Work out the finished part from the listing and answer in its coordinate system (mm). Face numbers are marked on the shaded views. Coordinates: 2 decimals unless noted, no trailing zeros. Write each loop counter-clockwise with the first axis right and the second up, starting at its lowest first coordinate (ties: lowest second). Pieces come first, ordered by that corner, then holes. Notation, with made-up numbers: (-13.75, -9.5) - (-0.75, -9.5) arc R10 ccw to (-0.75, -2.5) - close; hole circle Ø6 at (57.25, 21). An arc over 180 degrees is marked (long way). Use one line per item in the form item = value. Start each with the question number.
Item 1: Consider probe 1 along X at (y, z) = (1.1, -38) (3 decimals); probe 2 along Z at (x, y) = (1.5, 2.15); probe 3 along X at (y, z) = (2.2, -36.75). Determine where each line is inside the solid, lowest interval first.
Item 2: Determine the mould class of the marked faces 1, 2 and 3 for opening direction X: released by +X, released by -X, zero draft, split by the parting line, or undercut.
Item 3: A cutting plane is placed at D-D (x = 11). Write down the section's boundary in (y, z), then the cut area to 3 significant figures.
Item 4: A cutting plane is placed at A-A (x = 0). Write down the section's boundary in (y, z) (3 decimals).
Item 5: A cutting plane is placed at C-C (z = -38). Write down the section's boundary in (x, y) (3 decimals), then the cut area to 3 significant figures.
Item 6: A cutting plane is placed at B-B (y = 1.05). Write down the section's boundary in (x, z) (3 decimals).
Item 7: Given pin 1 (1.5 mm diameter, centred on x = 8, y = 2.5, fed in from +Z), flat-ended and moving along its own axis, determine where the tip first touches the part or whether it passes through.
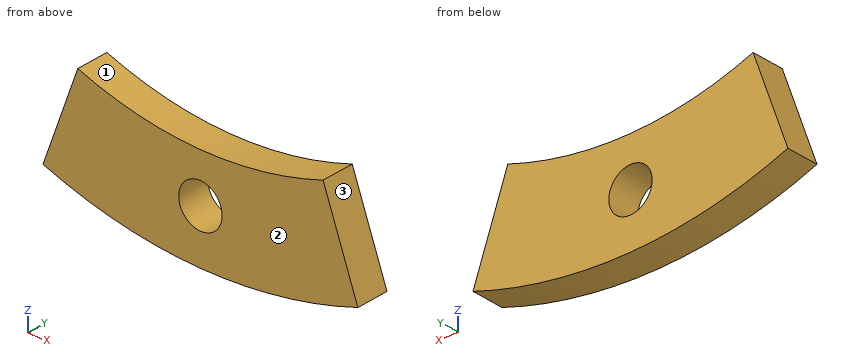
from build123d import *

# Parameters (mm, degrees)
SKETCH1_R               = 43
SKETCH1_R_2             = 33.5
BOSS_EXTRUDE1_DEPTH     = 3
CUT_EXTRUDE1_START      = -4
CUT_EXTRUDE1_DEPTH      = 5
SKETCH3_R               = 2.025
CUT_EXTRUDE2_DEPTH      = 1
CUT_EXTRUDE2_DEPTH_BACK = 4


with BuildPart() as part:
    # Sketch1 → Boss-Extrude1 (new body)
    with BuildSketch(Plane(origin=(0, 0, 0), x_dir=(1, 0, 0), z_dir=(0, 1, 0))):
        Circle(SKETCH1_R)
        Circle(SKETCH1_R_2, mode=Mode.SUBTRACT)
    extrude(amount=BOSS_EXTRUDE1_DEPTH)

    # Sketch2 → Cut-Extrude1 (cut)
    with BuildSketch(Plane(origin=(0, 3, 0), x_dir=(1, 0, 0), z_dir=(0, 1, 0)).offset(CUT_EXTRUDE1_START)):
        with BuildLine():
            Line((0, 0), (0, -52.31984462))
            ThreePointArc((0, -52.31984462), (51.524988618, -9.085245674), (17.894440756, 49.16457191))
            Line((17.894440756, 49.16457191), (0, 0))
        make_face()
    cut_extrude1 = extrude(amount=CUT_EXTRUDE1_DEPTH, mode=Mode.SUBTRACT)

    # Mirror1: Cut-Extrude1 across plane
    add(cut_extrude1.mirror(Plane(origin=(0, 0, 0), x_dir=(0, 0, 1), z_dir=(1, 0, 0))), mode=Mode.SUBTRACT)

    # Sketch3 → Cut-Extrude2 (cut, two sides)
    with BuildSketch(Plane(origin=(0, 3, 0), x_dir=(1, 0, 0), z_dir=(0, 1, 0))) as cut_extrude2_sk:
        with Locations((0, 38)):
            Circle(SKETCH3_R)
    extrude(amount=CUT_EXTRUDE2_DEPTH, mode=Mode.SUBTRACT)
    extrude(cut_extrude2_sk.sketch, amount=-CUT_EXTRUDE2_DEPTH_BACK, mode=Mode.SUBTRACT)


solid = part.part
Answer:
q1.probe_1 = -13.831 to -2.025, 2.025 to 13.831
q1.probe_2 = -42.97 to -39.36, -36.64 to -33.47
q1.probe_3 = -13.38 to -1.59, 1.59 to 13.38
q2.face_1 = undercut
q2.face_2 = zero draft
q2.face_3 = released by +X
q3.outline = (0, -41.57) - (3, -41.57) - (3, -31.64) - (0, -31.64) - close
q3.area = 29.8 mm²
q4.outline = (0, -43) - (3, -43) - (3, -40.025) - (0, -40.025) - close; (0, -35.975) - (3, -35.975) - (3, -33.5) - (0, -33.5) - close
q5.outline = (-13.831, 0) - (-2.025, 0) - (-2.025, 3) - (-13.831, 3) - close; (2.025, 0) - (13.831, 0) - (13.831, 3) - (2.025, 3) - close
q5.area = 70.8 mm²
q6.outline = (-14.707, -40.407) arc R43 ccw to (14.707, -40.407) - (11.458, -31.48) arc R33.5 cw to (-11.458, -31.48) - close; hole circle Ø4.05 at (0, -38)
q7.pin_1 = -32.34
